The listing builds one solid part. Answer for the finished solid, in the listing's coordinates (mm). A direction names the side the tool comes from. Round coordinates to 2 decimals unless told otherwise and drop trailing zeros. Write each loop counter-clockwise with the first axis right and the second up, starting at its lowest first coordinate (ties: lowest second). Pieces come first, ordered by that corner, then holes. Notation, with made-up numbers: (59.5, -34) -> (109.5, -34) arc R12 cw to (109.5, -17) -> close; hole circle Ø9 at (87, -30). An arc over 180 degrees is marked (long way). Write each question's results on one line, items separated by ' | '. Start each with the question number.
```python
from build123d import *

# Parameters (mm, degrees)
SKETCH1_R           = 9.525
SKETCH1_R_2         = 6.35
BOSS_EXTRUDE1_DEPTH = 66.675
BOSS_EXTRUDE2_DEPTH = 60.325


with BuildPart() as part:
    # Sketch1 → Boss-Extrude1 (new, symmetric)
    with BuildSketch(Plane(origin=(0, 0, 0), x_dir=(1, 0, 0), z_dir=(0, 1, 0))):
        with Locations(Location((0, 0, 0), (0, 0, 270))):
            Circle(SKETCH1_R)
        with Locations(Location((0, 0, 0), (0, 0, 270))):
            Circle(SKETCH1_R_2, mode=Mode.SUBTRACT)
    extrude(amount=BOSS_EXTRUDE1_DEPTH, both=True)

    # Sketch2 → Boss-Extrude2 (add, symmetric)
    with BuildSketch(Plane(origin=(0, 0, 0), x_dir=(1, 0, 0), z_dir=(0, 1, 0))):
        with BuildLine():
            Line((9.525, 0), (44.45, 0))
            Line((44.45, 0), (44.45, -12.7))
            Line((44.45, -12.7), (-44.45, -12.7))
            Line((-44.45, -12.7), (-44.45, 0))
            Line((-44.45, 0), (-9.525, 0))
            ThreePointArc((-9.525, 0), (0, -9.525), (9.525, 0))
        make_face()
    extrude(amount=BOSS_EXTRUDE2_DEPTH, both=True)


solid = part.part
```
Q1. The part is cut by section D-D, the plane x = -19. Write down the section's boundary in (y, z) (3 decimals), then the cut area to 3 significant figures.
Q2. Each of these flat-tipped pins is pushed along its axis until it touches: pin 1 (10 mm diameter, centred on y = -25.5, z = -3, fed in from +X); pin 2 (2 mm diameter, centred on x = -2, y = 21.5, fed in from -Z); pin 3 (10 mm diameter, centred on x = 20.5, z = 7, fed in from +Y) (3 decimals); pin 4 (2 mm diameter, centred on x = -17, z = 3.5, fed in from -Y) (3 decimals). Where does it stop, or does it pass through?
Q3. The part is cut by section A-A, the plane x = 0. Write down the section's boundary in (y, z) (3 decimals), then the cut area to 3 significant figures.
Q4. The part is cut by section B-B, the plane y = -40. Write down the section's boundary in (x, z) (3 decimals), then the cut area to 3 significant figures.
Q5. Determine the mould class of faces 1 (the flat face through (-27, 1, 0)), 2 (the flat face through (1, 1, 12.7)), 3 (the cylindrical face through (-3.86, -0.93, -5.04)), 4 (the flat face through (1, 60.325, 10)) for opening direction Z: pulls with the +Z half, pulls with the -Z half, needs draft (parallel to the pull), parting line crosses it, or undercut.
Q6. The part is cut by section C-C, the plane z = -5. Write down the section's boundary in (x, y) (3 decimals), then the cut area to 3 significant figures.
Q7. For faces 5 (the flat face through (27, 1, 0)), 6 (the flat face through (-6.2, 66.675, 2)), 7 (the flat face through (1, -60.325, 10)), determine the directions among +Z, -Z, +X, -X, +Y, -Y from which every point of the face is accessible in a straight line to the end or side of a thin tool.
Q8. Find the intervals of material crossed by line 1 (Y direction, x = 20, z = 5.25) (3 decimals); line 2 (Z direction, x = 25.5, y = -53); line 3 (X direction, y = 58.5, z = 3.5), in increasing order.
Answers follow:
1) outline: (-60.325, 0) -> (60.325, 0) -> (60.325, 12.7) -> (-60.325, 12.7) -> close | area: 1,530 mm^2
2) pin 1: x = 44.45 | pin 2: z = -9.47 | pin 3: y = 60.325 | pin 4: y = -60.325
3) outline: (-66.675, -9.525) -> (66.675, -9.525) -> (66.675, -6.35) -> (-66.675, -6.35) -> close; (-66.675, 6.35) -> (66.675, 6.35) -> (66.675, 9.525) -> (60.325, 9.525) -> (60.325, 12.7) -> (-60.325, 12.7) -> (-60.325, 9.525) -> (-66.675, 9.525) -> close | area: 1,230 mm^2
4) outline: (-44.45, 0) -> (-9.525, 0) arc R9.525 ccw to (9.525, 0) -> (44.45, 0) -> (44.45, 12.7) -> (-44.45, 12.7) -> close; hole circle Ø12.7 at (0, 0) | area: 1,140 mm^2
5) face 1: pulls with the -Z half | face 2: pulls with the +Z half | face 3: undercut | face 4: needs draft
6) outline: (-8.107, -66.675) -> (-3.914, -66.675) -> (-3.914, 66.675) -> (-8.107, 66.675) -> close; (3.914, -66.675) -> (8.107, -66.675) -> (8.107, 66.675) -> (3.914, 66.675) -> close | area: 1,120 mm^2
7) face 5: -Z, +X, +Y, -Y | face 6: +Z, -Z, +X, -X, +Y | face 7: +Z, -Y
8) line 1: -60.325 to 60.325 | line 2: 0 to 12.7 | line 3: -44.45 to -5.3, 5.3 to 44.45
